Could you check a few things on this model? Use its own coordinates, in mm. A direction names the side the tool comes from. Coordinates: 2 decimals unless noted, no trailing zeros. Write each loop counter-clockwise with the first axis right and the second up, starting at its lowest first coordinate (ties: lowest second). Pieces come first, ordered by that corner, then holes. Notation, with made-up numbers: M 21,-26 L 79,-26 A10 ccw 79,-10 Z; hole C 44.5,6 d8. An arc over 180 degrees is marked long. Answer as CSV lines item,"result". Start each with the question number.
Item 1: Suppose I cut it at C-C, the plane y = -9. Write out the boundary of the cut face in (x, z), and give its area (3 significant figures).
Item 2: Suppose I cut it at D-D, the plane y = 3.75. Write out the boundary of the cut face in (x, z), and give its area (3 significant figures).
Item 3: If I drill on line 1 along X through (y, z) = (4, 0.3); line 2 along X through (y, z) = (-9.75, -0.3); line 3 along Y through (x, z) = (19, 0.1), over which ranges is the centre line in solid material (lowest first)? Write a range as [from, to].
Item 4: I'm going to push a flat-ended pin straight in: P1, Ø1.5, axis at x = 65.5, z = -1, coming from the -Y side. Where does the tip first touch, or does it pass through?
Item 5: On a 3-axis mill with a long thin cutter (end or side, diameter ignored), from which of +Z, -Z, +X, -X, +Y, -Y can I reach the whole of each face in a straight line? I mean faces 1 (the cylindrical face through (97.535, -11.787, -1.748)), 2 (the flat face through (95, -10, 0)), 3 (the flat face through (95, 5, 0)). Say none if no direction works.
Item 6: Suppose I cut it at A-A, the plane z = 1.5. Write out the boundary of the cut face in (x, y), and give its area (3 significant figures).
```python
from build123d import *

# Parameters (mm, degrees)
F1_DEPTH = 2.5
F2_R     = 2.49999


# Not quite as in the source:
# - a fillet or chamfer is up to 0.001 mm smaller than in the source, because OpenCascade refuses the exact size


with BuildPart() as f1:
    # F0 (on Top) → F1 (new body, symmetric)
    with BuildSketch(Plane.XY):
        Polygon((95, 7.5), (0, 7.5), (0, -7.5), (95, -7.5), (95, -12.5), (100, -12.5), (100, 2.5), (95, 2.5), align=None)
    extrude(amount=F1_DEPTH, both=True)

    # F2 (radius 2.5 in the source; OpenCascade refuses exactly that, so slightly less here)
    f2_edges = [f1.edges().sort_by_distance(p)[0] for p in [
        (97.5, -12.5, 2.5),
        (97.5, -12.5, -2.5),
        (47.5, 7.5, 2.5),
        (47.5, 7.5, -2.5),
    ]]
    fillet(f2_edges, radius=F2_R)


solid = f1.part
```
Ans:
1,outline,"M 95,-2.5 L 100,-2.5 L 100,2.5 L 95,2.5 Z"
1,area,"25.0 mm^2"
2,outline,"M 0,-2.5 L 95,-2.5 L 95,2.5 L 0,2.5 Z"
2,area,"475 mm^2"
3,line 1,"x = [0, 95]"
3,line 2,"x = [95, 100]"
3,line 3,"y = [-7.5, 7.5]"
4,P1,"stops at y = -7.5"
5,face 1,"-Z, +X, -X, -Y"
5,face 2,"+Z, -Z, -X, -Y"
5,face 3,"+Z, -Z, +X, +Y"
6,outline,"M 0,-7.5 L 95,-7.5 L 95,-12 L 100,-12 L 100,2.5 L 95,2.5 L 95,7 L 0,7 Z"
6,area,"1,450 mm^2"
